from build123d import *

# Parameters (mm, degrees)
SKETCH1_R           = 7.5
BOSS_EXTRUDE1_DEPTH = 130
SKETCH2_R           = 10
BOSS_EXTRUDE2_DEPTH = 5
BOSS_EXTRUDE3_START = 10
SKETCH3_R           = 7.5
BOSS_EXTRUDE3_DEPTH = 10
CUT_EXTRUDE1_START  = -80
CUT_EXTRUDE1_DEPTH  = 80
BOSS_EXTRUDE4_DEPTH = 1.5


with BuildPart() as part:
    # Sketch1 → Boss-Extrude1 (new body)
    with BuildSketch(Plane.XY):
        Circle(SKETCH1_R)
    extrude(amount=-BOSS_EXTRUDE1_DEPTH)

    # Sketch2 → Boss-Extrude2 (add)
    with BuildSketch(Plane.XY):
        Circle(SKETCH2_R)
    extrude(amount=BOSS_EXTRUDE2_DEPTH)

    # Sketch3 → Boss-Extrude3 (add)
    with BuildSketch(Plane.XY.offset(5).offset(BOSS_EXTRUDE3_START)):
        Circle(SKETCH3_R)
    extrude(amount=-BOSS_EXTRUDE3_DEPTH)

    # Sketch4 → Cut-Extrude1 (cut)
    with BuildSketch(Plane(origin=(0, 0, -130), x_dir=(-1, 0, 0), z_dir=(0, 0, -1)).offset(CUT_EXTRUDE1_START)):
        with BuildLine():
            Line((-6.5, 3.741657387), (-6.5, -3.741657387))
            ThreePointArc((-6.5, -3.741657387), (-7.5, 0), (-6.5, 3.741657387))
        make_face()
        with BuildLine():
            Line((6.5, 3.741657387), (6.5, -3.741657387))
            ThreePointArc((6.5, -3.741657387), (7.5, 0), (6.5, 3.741657387))
        make_face()
    extrude(amount=CUT_EXTRUDE1_DEPTH, mode=Mode.SUBTRACT)

    # Sketch6 → Boss-Extrude4 (add, symmetric)
    with BuildSketch(Plane(origin=(0, 0, 0), x_dir=(1, 0, 0), z_dir=(0, 1, 0))):
        with BuildLine():
            Line((-6, -18), (-6, -15))
            Line((-6, -15), (6, -15))
            Line((6, -15), (6, -18))
            ThreePointArc((6, -18), (0, -24), (-6, -18))
        make_face()
    extrude(amount=BOSS_EXTRUDE4_DEPTH, both=True)


solid = part.part
Source: CAD feature listing. Evaluate the final solid. Frame: model axes, mm. A direction names the side the tool comes from. Round coordinates to 2 decimals unless told otherwise and drop trailing zeros. Loops run counter-clockwise (first coordinate to the right, second up) from the corner with the lowest first, then second, coordinate; pieces in that order, holes last. Notation, with made-up numbers: (34.5, 24.25) - (59.5, 24.25) arc R16 ccw to (59.5, 39.25) - close; hole circle Ø4 at (0.5, 49.5). An arc over 180 degrees is marked (long way). Write item = value, one per line. Start each with the question number.
(1) Ray query, line 1 along Z through (x, y) = (6, -5.75); line 2 along X through (y, z) = (-1, -81); line 3 along Z through (x, y) = (-1, -1.75). Return the intervals inside material, ascending. Write a range as from..to.
(2) Set-up query: faces 1 (the face through (0, -1.5, 18)), 2 (the face through (0, 1.5, 18)), 3 (the face through (-6.5, 0, -89)). Return all of +Z, -Z, +X, -X, +Y, -Y with unobstructed straight access to the full face (end or side cutting, diameter ignored); none if empty.
(3) Section query D-D, the plane y = -6. Output: boundary loops of the cut face in (x, z), plus the area to 3 significant figures.
(4) Section query A-A, the plane y = 0. Output: boundary loops of the cut face in (x, z), plus the area to 3 significant figures.
(5) Section query B-B, the plane x = 4. Output: boundary loops of the cut face in (y, z).
(6) Pin query (flat end, axial travel): pin 1 (1.5 mm diameter, centred on y = 0.5, z = 16.5, fed in from +X); pin 2 (8 mm diameter, centred on y = 1.5, z = -98.5, fed in from -X); pin 3 (2 mm diameter, centred on x = -3, z = -31, fed in from +Y). Return the tip coordinate at first contact, or that it passes through.
(7) Section query C-C, the plane z = -41. Output: boundary loops of the cut face in (x, y), plus the area to 3 significant figures.
Conclusion:
q1.line_1 = 0..5
q1.line_2 = -6.5..6.5
q1.line_3 = -130..15
q2.face_1 = +Z, +X, -X, -Y
q2.face_2 = +Z, +X, -X, +Y
q2.face_3 = -Z, -X, +Y, -Y
q3.outline = (-8, 0) - (-4.5, 0) - (-4.5, -130) - (4.5, -130) - (4.5, 0) - (8, 0) - (8, 5) - (4.5, 5) - (4.5, 15) - (-4.5, 15) - (-4.5, 5) - (-8, 5) - close
q3.area = 1,340 mm2
q4.outline = (-10, 0) - (-7.5, 0) - (-7.5, -50) - (-6.5, -50) - (-6.5, -130) - (6.5, -130) - (6.5, -50) - (7.5, -50) - (7.5, 0) - (10, 0) - (10, 5) - (7.5, 5) - (7.5, 15) - (6, 15) - (6, 18) arc R6 ccw to (-6, 18) - (-6, 15) - (-7.5, 15) - (-7.5, 5) - (-10, 5) - close
q4.area = 2,130 mm2
q5.outline = (-9.17, 0) - (-6.34, 0) - (-6.34, -130) - (6.34, -130) - (6.34, 0) - (9.17, 0) - (9.17, 5) - (6.34, 5) - (6.34, 15) - (1.5, 15) - (1.5, 22.47) - (-1.5, 22.47) - (-1.5, 15) - (-6.34, 15) - (-6.34, 5) - (-9.17, 5) - close
q6.pin_1 = 6
q6.pin_2 = -6.5
q6.pin_3 = 7.23
q7.outline = circle Ø15 at (0, 0)
q7.area = 177 mm2
